Design review of the part built by this model. Coordinates are the model's own, in mm. A direction names the side the tool comes from. Give positions to 0.01 mm unless a question says otherwise; leave off trailing zeros. Loops run counter-clockwise (first coordinate to the right, second up) from the corner with the lowest first, then second, coordinate; pieces in that order, holes last. Notation, with made-up numbers: M 34.5,57.25 L 81.5,57.25 A17 cw 81.5,73.25 Z; hole C 14,38.5 d3. An arc over 180 degrees is marked long. Use CSV: the item, a comma, the result in double quotes.
from build123d import *

# Parameters (mm, degrees)
F0_W     = 20
F0_H     = 50
F1_DEPTH = 5
F2_W     = 5
F2_H     = 8
F3_DEPTH = 5
F4_R     = 1
F6_D     = 6.6
F7_W     = 20
F7_H     = 5
F8_DEPTH = 30
F9_R     = 1
F11_D    = 6.6
F13_D    = 5.5
F14_R    = 2.5


with BuildPart() as f1:
    # F0 (on Top) → F1 (new body)
    with BuildSketch(Plane.XY):
        Rectangle(F0_W, F0_H)
    extrude(amount=F1_DEPTH)

    # F2 (on face) → F3 (join)
    with BuildSketch(Plane(origin=(0, 0, 0), x_dir=(1, 0, 0), z_dir=(0, 0, -1))):
        with Locations((0, -20)):
            Rectangle(F2_W, F2_H)
        with Locations((0, 5)):
            Rectangle(F2_W, F2_H)
    extrude(amount=F3_DEPTH)

    # F4
    f4_edges = [f1.edges().sort_by_distance(p)[0] for p in [
        (2.5, 20, -5),
        (-2.5, 20, -5),
        (0, 24, -5),
        (0, 16, -5),
        (0, -1, -5),
        (-2.5, -5, -5),
        (0, -9, -5),
        (2.5, -5, -5),
    ]]
    fillet(f4_edges, radius=F4_R)

    # F6 (through all)
    with Locations(Plane(origin=(0, 0, 0), x_dir=(1, 0, 0), z_dir=(0, 0, -1))):
        with Locations((0, -10)):
            Hole(F6_D / 2)

    # F7 (on face) → F8 (join)
    with BuildSketch(Plane.XY.offset(5)):
        with Locations((0, -7.5)):
            Rectangle(F7_W, F7_H)
    extrude(amount=F8_DEPTH)

    # F9
    f9_edges = [f1.edges().sort_by_distance(p)[0] for p in [
        (10, -7.5, 35),
        (-10, -7.5, 35),
    ]]
    fillet(f9_edges, radius=F9_R)

    # F11 (through all)
    with Locations(Plane.XZ.offset(10)):
        with Locations((0, 20)):
            Hole(F11_D / 2)

    # F13 (through all)
    with Locations(Plane.XY.offset(5)):
        with Locations((0, -17.5)):
            Hole(F13_D / 2)

    # F14
    f14_edges = [f1.edges().sort_by_distance(p)[0] for p in [
        (0, 25, 5),
        (0, -25, 5),
    ]]
    fillet(f14_edges, radius=F14_R)


solid = f1.part
(1) We need section C-C on y = -17.5. State the section outline as (x, z) points.
A:
outline,"M -10,0 L -2.75,0 L -2.75,5 L -10,5 Z; M 2.75,0 L 10,0 L 10,5 L 2.75,5 Z"
(2) Clearance check with flat-ended pins moving along their axes: P1, Ø6, axis at x = -1, y = -18.5, coming from the +Z side; P2, Ø3, axis at x = 0.5, z = -2.5, coming from the +Y side; P3, Ø2, axis at y = 18.5, z = -1.5, coming from the +X side. State where each tip first meets the part, or that it passes through.
A:
P1,"z = 5"
P2,"y = 24"
P3,"x = 2.5"
(3) The part is to be moulded in two halves that separate along Z. For faces 1 (the cylindrical face through (0.72, -7.47, 16.78)), 2 (the flat face through (-2, -15, 5)), 3 (the flat face through (0, 16, -2)), say which applies: released by +Z, released by -Z, zero draft, split by the parting line, or undercut.
A:
face 1,"undercut"
face 2,"released by +Z"
face 3,"zero draft"
(4) We need section B-B on x = 0. Count the separate pieces of the cut face and the enclosed holes in it, then the cut area to 3 significant figures.
A:
separate pieces,"4"
enclosed holes,"0"
area,"383 mm²"
(5) Wall thickness on line 1 along Y through (x, z) = (0, 1.7); line 2 along Z through (x, y) = (0, -7.85); line 3 along Z through (x, y) = (3.75, 17.5): over which ranges is each line inside the solid? List them lowest first. Write a range as [from, to].
A:
line 1,"[-25, -20.25], [-14.75, 6.7], [13.3, 25]"
line 2,"[-5, 16.7], [23.3, 35]"
line 3,"[0, 5]"
(6) We need section D-D on x = -4. State the section outline as (y, z) points, then the cut area to 3 significant figures.
A:
outline,"M -25,0 L 25,0 L 25,2.5 A2.5 ccw 22.5,5 L -5,5 L -5,35 L -10,35 L -10,5 L -22.5,5 A2.5 ccw -25,2.5 Z"
area,"397 mm²"
(7) We need section A-A on z = -1.5. State the section outline as (x, y) points.
A:
outline,"M -2.5,-9 L 2.5,-9 L 2.5,-1 L -2.5,-1 Z; M -2.5,16 L 2.5,16 L 2.5,24 L -2.5,24 Z"
(8) Machinability: for faces 4 (the flat face through (2.5, 20, -2)), 5 (the flat face through (0, -9, -2)), 6 (the flat face through (0, -1, -2)), 7 (the flat face through (0, 24, -2)), which of the approach directions +Z, -Z, +X, -X, +Y, -Y give a long, thin tool a straight path to every point of the face, cutting with its end or side? Answer none if there is none.
A:
face 4,"-Z, +X, +Y, -Y"
face 5,"-Z, +X, -X, -Y"
face 6,"-Z, +X, -X"
face 7,"-Z, +X, -X, +Y"
